The listing builds one solid part. Answer for the finished solid, in the listing's coordinates (mm). Face numbers are marked on the shaded views. A direction names the side the tool comes from. Give positions to 0.01 mm unless a question says otherwise; leave off trailing zeros. Order: outer loops, then holes, each group sorted by start corner. A loop starts at its lowest first (then second) coordinate and runs counter-clockwise, first axis right, second up. Notation, with made-up numbers: M 28.5,-39.5 L 72.5,-39.5 A14 cw 72.5,-14.5 Z; hole C 6,31.5 d8. An arc over 180 degrees is marked long. Answer as a JSON object with one key per item and string values. Group by question number.
```python
from build123d import *

# Parameters (mm, degrees)
SKETCH_1_R               = 5.3
SKETCH_1_R_2             = 11.1
EXTRUDE_1_DEPTH          = 7
SKETCH_2_R               = 11.3
SKETCH_2_W               = 42.2
SKETCH_2_H               = 42.2
CUT_EXTRUDE_1_DEPTH      = 2
SKETCH_3_R               = 1.6
CUT_EXTRUDE_2_DEPTH      = 99.783854956
EXTRUDE_2_DEPTH          = 21.9
CUT_EXTRUDE_3_DEPTH      = 96.645438992
CUT_EXTRUDE_4_DEPTH      = 89.767730623
CUT_EXTRUDE_4_DEPTH_BACK = 10
CUT_EXTRUDE_5_DEPTH      = 102.058695816
SKETCH_8_R               = 1.6
SKETCH_8_W               = 41.679602286
SKETCH_8_H               = 26.376779249
CUT_EXTRUDE_6_DEPTH      = 89.386707145
SKETCH_9_R               = 3
CUT_EXTRUDE_7_DEPTH      = 3
CUT_EXTRUDE_8_DEPTH      = 3
SKETCH_11_W              = 44
SKETCH_11_H              = 5
CUT_EXTRUDE_9_DEPTH      = 89.495536611
SKETCH_12_W              = 37.71360908
SKETCH_12_H              = 40.060480483
CUT_EXTRUDE_11_DEPTH     = 5
SKETCH_13_W              = 8.835151958
SKETCH_13_H              = 10.520362882
CUT_EXTRUDE_12_DEPTH     = 87.463055694


with BuildPart() as part:
    # Sketch 1 → Extrude 1 (new body)
    with BuildSketch(Plane.XY):
        Polygon((-68.5, 26), (-24.5, 26), (-24.5, 71), (-19.5, 71), (-19.5, 26), (-19.5, 25.5), (14.5, 25.5), (14.5, -25), (-68.5, -25), align=None)
        Circle(SKETCH_1_R, mode=Mode.SUBTRACT)
        with Locations((-45.5, -2)):
            Circle(SKETCH_1_R_2, mode=Mode.SUBTRACT)
    extrude(amount=EXTRUDE_1_DEPTH)

    # Sketch 2 → Cut-Extrude 1 (cut)
    with BuildSketch(Plane.XY.offset(7)):
        Circle(SKETCH_2_R)
        with Locations((-45.6, -2)):
            Rectangle(SKETCH_2_W, SKETCH_2_H)
    extrude(amount=-CUT_EXTRUDE_1_DEPTH, mode=Mode.SUBTRACT)

    # Sketch 3 → Cut-Extrude 2 (cut, through all)
    with BuildSketch(Plane.XY.offset(5)):
        with Locations((-61, 13.5)):
            Circle(SKETCH_3_R)
        with Locations(Location((-30, 13.5, 0), (0, 0, 180))):
            Circle(SKETCH_3_R)
        with Locations((-30, -17.5)):
            Circle(SKETCH_3_R)
        with Locations(Location((-61, -17.5, 0), (0, 0, 180))):
            Circle(SKETCH_3_R)
        with Locations((5.656854249, 5.656854249)):
            Circle(SKETCH_3_R)
        with Locations((-5.656854249, 5.656854249)):
            Circle(SKETCH_3_R)
        with Locations((5.656854249, -5.656854249)):
            Circle(SKETCH_3_R)
        with Locations((-5.656854249, -5.656854249)):
            Circle(SKETCH_3_R)
    extrude(amount=-CUT_EXTRUDE_2_DEPTH, mode=Mode.SUBTRACT)

    # Sketch 4 → Extrude 2 (add)
    with BuildSketch(Plane.XY.offset(7)):
        Polygon((-19.5, 68.4214033), (-24.5, 71), (-24.5, 26), (-68.5, 26), (-68.5, 19.1), (-24.5, 19.1), (-24.5, -14.479637118), (-11.3, -14.479637118), (-11.3, 22.5), (14.5, 22.5), (14.5, 25.5), (-19.5, 25.5), align=None)
    extrude(amount=EXTRUDE_2_DEPTH)

    # Sketch 5 → Cut-Extrude 3 (cut, through all)
    with BuildSketch(Plane(origin=(-11.3, 0, 0), x_dir=(0, 0, -1), z_dir=(1, 0, 0))):
        Polygon((-28.9, 19.1), (-28.9, -14.479637118), (-7, -14.479637118), (-6.982294127, -14.420838609), align=None)
    extrude(amount=-CUT_EXTRUDE_3_DEPTH, mode=Mode.SUBTRACT)

    # Sketch 6 → Cut-Extrude 4 (cut, two sides: drawn at the far end of the back side and taken through both)
    with BuildSketch(Plane.XZ.offset(-22.5).offset(-CUT_EXTRUDE_4_DEPTH_BACK)):
        Polygon((-68.5, 7), (-24.5, 28.9), (-68.5, 28.9), align=None)
        Polygon((-19.5, 28.9), (14.5, 7), (14.5, 28.9), align=None)
    extrude(amount=CUT_EXTRUDE_4_DEPTH + CUT_EXTRUDE_4_DEPTH_BACK, mode=Mode.SUBTRACT)

    # Sketch 7 → Cut-Extrude 5 (cut, through all)
    with BuildSketch(Plane.XY.offset(7)):
        with BuildLine():
            Line((-13.15, -14.479637118), (-11.3, -14.479637118))
            Line((-11.3, -14.479637118), (-0.0261596, -14.499976403))
            ThreePointArc((-0.0261596, -14.499976403), (10.243795337, -10.262292975), (14.5, 0))
            Line((14.5, 0), (21.147002499, 0))
            Line((21.147002499, 0), (22.768629324, -44.459429771))
            Line((22.768629324, -44.459429771), (-13.15, -44.459429771))
            Line((-13.15, -44.459429771), (-13.15, -14.479637118))
        make_face()
    extrude(amount=-CUT_EXTRUDE_5_DEPTH, mode=Mode.SUBTRACT)

    # Sketch 8 → Cut-Extrude 6 (cut, through all)
    with BuildSketch(Plane.ZY.offset(24.5)):
        with Locations(Location((19, 28.5, 0), (0, 0, 270))):
            Circle(SKETCH_8_R)
        with Locations(Location((19, 43.5, 0), (0, 0, 270))):
            Circle(SKETCH_8_R)
        with Locations(Location((9, 28.5, 0), (0, 0, 270))):
            Circle(SKETCH_8_R)
        with Locations(Location((9, 43.5, 0), (0, 0, 270))):
            Circle(SKETCH_8_R)
        with Locations((14.868313548, 61.188389625)):
            Rectangle(SKETCH_8_W, SKETCH_8_H)
        with BuildLine():
            Line((15.75, 37.75), (15.75, 34.25))
            ThreePointArc((15.75, 34.25), (14, 32.5), (12.25, 34.25))
            Line((12.25, 34.25), (12.25, 37.75))
            ThreePointArc((12.25, 37.75), (14, 39.5), (15.75, 37.75))
        make_face()
    extrude(amount=-CUT_EXTRUDE_6_DEPTH, mode=Mode.SUBTRACT)

    # Sketch 9 → Cut-Extrude 7 (cut)
    with BuildSketch(Plane.ZY.offset(24.5)):
        with Locations(Location((9, 43.5, 0), (0, 0, 270))):
            Circle(SKETCH_9_R)
        with Locations(Location((19, 43.5, 0), (0, 0, 270))):
            Circle(SKETCH_9_R)
        with Locations(Location((9, 28.5, 0), (0, 0, 270))):
            Circle(SKETCH_9_R)
        with Locations(Location((19, 28.5, 0), (0, 0, 270))):
            Circle(SKETCH_9_R)
    extrude(amount=-CUT_EXTRUDE_7_DEPTH, mode=Mode.SUBTRACT)

    # Sketch 10 → Cut-Extrude 8 (cut)
    with BuildSketch(Plane(origin=(-19.5, 0, 0), x_dir=(0, 0, -1), z_dir=(1, 0, 0))):
        with BuildLine():
            Line((-11, 37.75), (-11, 34.25))
            ThreePointArc((-11, 34.25), (-14, 31.25), (-17, 34.25))
            Line((-17, 34.25), (-17, 37.75))
            ThreePointArc((-17, 37.75), (-14, 40.75), (-11, 37.75))
        make_face()
    extrude(amount=-CUT_EXTRUDE_8_DEPTH, mode=Mode.SUBTRACT)

    # Sketch 11 → Cut-Extrude 9 (cut, through all)
    with BuildSketch(Plane(origin=(0, 0, 0), x_dir=(-1, 0, 0), z_dir=(0, 0, -1))):
        with Locations((46.5, 23.5)):
            Rectangle(SKETCH_11_W, SKETCH_11_H)
    extrude(amount=-CUT_EXTRUDE_9_DEPTH, mode=Mode.SUBTRACT)

    # Sketch 12 → Cut-Extrude 11 (cut)
    with BuildSketch(Plane(origin=(-11.3, 0, 0), x_dir=(0, 0, -1), z_dir=(1, 0, 0))):
        with Locations((-25.85680454, 2.469759758)):
            Rectangle(SKETCH_12_W, SKETCH_12_H)
    extrude(amount=-CUT_EXTRUDE_11_DEPTH, mode=Mode.SUBTRACT)

    # Sketch 13 → Cut-Extrude 12 (cut, through all)
    with BuildSketch(Plane.XY.offset(7)):
        with Locations((-17.567575979, -19.739818559)):
            Rectangle(SKETCH_13_W, SKETCH_13_H)
    extrude(amount=-CUT_EXTRUDE_12_DEPTH, mode=Mode.SUBTRACT)


solid = part.part
```
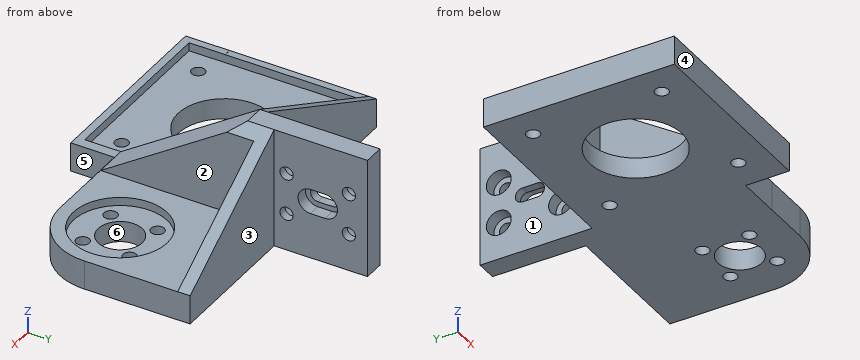
Item 1: A tool of negligible diameter and unlimited length cuts with its end or side. For the marked faces 1, 2 and 3, from which of +Z, -Z, +X, -X, +Y, -Y can it reach the whole face along a straight path? Write none if from no direction.
Item 2: Section B-B (x = -2) is taken. Determine the outline of the cut face in (y, z), and give its area (3 significant figures).
Item 3: Section C-C (z = 19) is taken. Determine the outline of the cut face in (x, y), and give its area (3 significant figures).
Item 4: Flat-ended cylindrical pins translate along their axes: P1, Ø3.5, axis at y = -19.5, z = 3.5, coming from the +X side; P2, Ø8, axis at x = -35, z = 24, coming from the +Y side; P3, Ø5, axis at y = -6.5, z = 6, coming from the +X side. Find the tip coordinate at first contact, or state that the pin passes through.
Item 5: Consider probe 1 along Y at (x, z) = (-61, 2.4); probe 2 along Z at (x, y) = (-20.4, 43.5); probe 3 along Y at (x, z) = (0, 6.05). Determine where each line is inside the solid, lowest interval first. Write a range as from..to.
Item 6: Section A-A (y = -2) is taken. Determine the outline of the cut face in (x, z).
Item 7: Determine the mould class of the marked faces 4, 5 and 6 for opening direction Y: released by +Y, released by -Y, zero draft, split by the parting line, or undercut.
Item 8: Section D-D (x = -61) is taken. Determine the outline of the cut face in (y, z), and give its area (3 significant figures).
Values found:
{
 "1": {"face 1": "+Z, -Z, -X, +Y", "face 2": "+Z, +X, -Y", "face 3": "+Z, -Z, +X, +Y"},
 "2": {"outline": "M -14.5,0 L -4.91,0 L -4.91,5 L -11.12,5 L -11.12,7 L -14.5,7 Z; M 4.91,0 L 25.5,0 L 25.5,17.63 L 22.5,17.63 L 22.5,7 L 11.12,7 L 11.12,5 L 4.91,5 Z", "area": "218 mm^2"},
 "3": {"outline": "M -44.39,19.1 L -24.5,19.1 L -24.5,3.96 L -16.3,3.96 L -16.3,22.5 L -4.13,22.5 L -4.13,25.5 L -19.5,25.5 L -19.5,26.9 L -21.5,26.9 L -21.5,25.5 L -24.5,25.5 L -24.5,21 L -44.39,21 Z; M -24.5,31.5 L -21.5,31.5 L -21.5,30.1 L -19.5,30.1 L -19.5,41.9 L -21.5,41.9 L -21.5,40.5 L -24.5,40.5 Z; M -24.5,46.5 L -21.5,46.5 L -21.5,45.1 L -19.5,45.1 L -19.5,48 L -24.5,48 Z", "area": "315 mm^2"},
 "4": {"P1": "stops at x = -21.99", "P2": "stops at y = 21", "P3": "stops at x = 13.94"},
 "5": {"probe 1": "y = -25..-19.1, -15.9..11.9, 15.1..21", "probe 2": "z = 0..7.4, 10.6..17.4, 20.6..28.9", "probe 3": "y = -14.5..-11.3, 11.3..25.5"},
 "6": {"outline": "M -68.5,0 L -56.6,0 L -56.6,5 L -66.7,5 L -66.7,7 L -68.5,7 Z; M -34.4,0 L -4.91,0 L -4.91,5 L -11.12,5 L -11.12,7 L -16.3,7 L -16.3,15.1 L -24.5,15.1 L -24.5,5 L -34.4,5 Z; M 4.91,0 L 14.36,0 L 14.36,7 L 11.12,7 L 11.12,5 L 4.91,5 Z"},
 "7": {"face 4": "released by -Y", "face 5": "zero draft", "face 6": "undercut"},
 "8": {"outline": "M -25,0 L -19.1,0 L -19.1,5 L -23.1,5 L -23.1,7 L -25,7 Z; M -15.9,0 L 11.9,0 L 11.9,5 L -15.9,5 Z; M 15.1,0 L 21,0 L 21,10.73 L 19.1,10.73 L 19.1,5 L 15.1,5 Z", "area": "213 mm^2"}
}
